Could you check a few things on this drawing? It's one solid part, dimensions in mm from its lowest x, y, z. A direction names the side the tool comes from. Round coordinates to 2 decimals unless told otherwise and drop trailing zeros. Loops run counter-clockwise (first coordinate to the right, second up) from the corner with the lowest first, then second, coordinate; pieces in that order, holes last. Notation, with made-up numbers: (9.25, 29) -> (54.25, 29) arc R12 ccw to (54.25, 50) -> close; hole circle Ø6 at (18, -11). An arc over 180 degrees is marked (long way). Put each result on its own line as item: value. Start each with the question number.
1. Imagine slicing it at A-A, the plane y = 44.5. Please give me the cut outline in (x, z), and give its area (3 significant figures).
2. I need wall thicknesses on line 1 (Y direction, x = 4.75, z = 10); line 2 (Z direction, x = 6.75, y = 17); line 3 (X direction, y = 20, z = 9). Which ranges of each line are inside material? Lowest first, please. Write a range as [from, to].
3. Which directions (+Z, -Z, +X, -X, +Y, -Y) give clear straight access to the entire face, cutting with the end or side of a thin tool? Please do the marked faces 1 and 2.
4. I'm going to push flat-ended pins straight in: P1, Ø3, axis at x = 12.5, y = 25, coming from the +Z side; P2, Ø6.5, axis at x = 8.5, z = 4, coming from the -Y side; P3, Ø2, axis at y = 10, z = 9.5, coming from the +X side; P4, Ø1, axis at x = 12, z = 4.5, coming from the -Y side. Where does each tip first touch, or does it pass through?
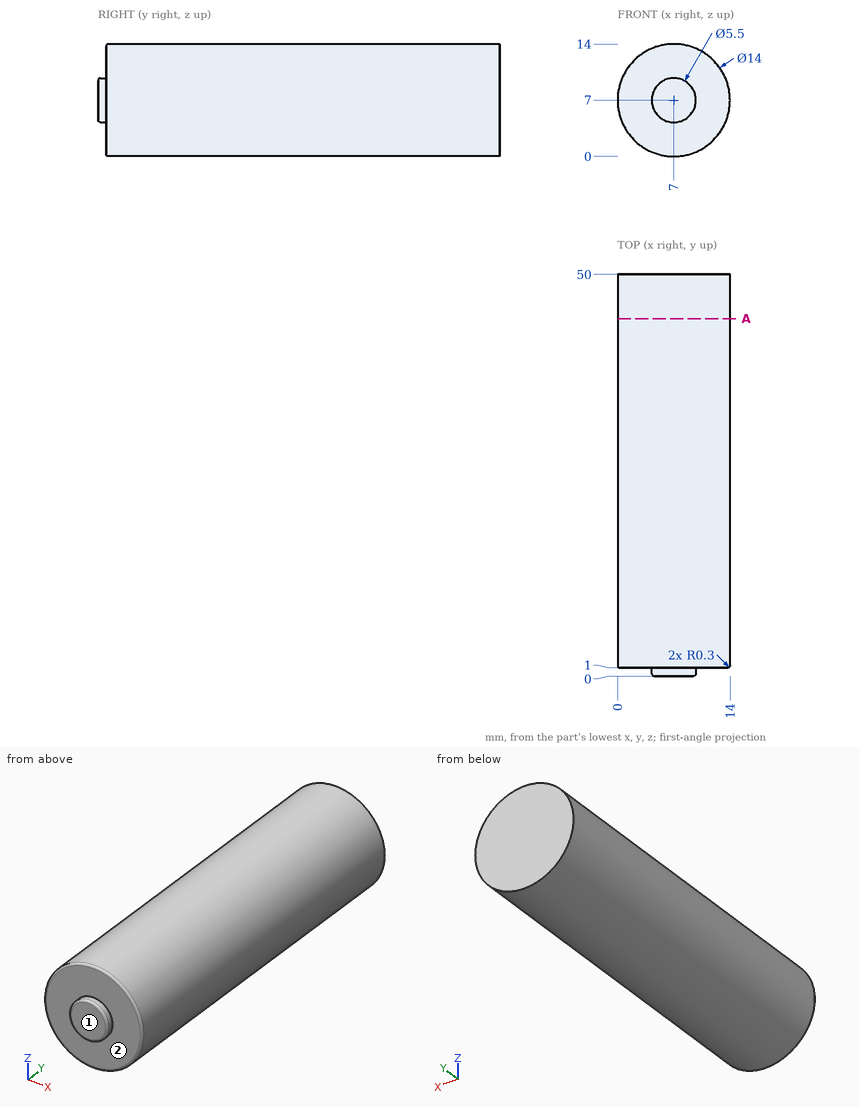
Entries:
1. outline: circle Ø14 at (7, 7)
1. area: 154 mm^2
2. line 1: [1, 50]
2. line 2: [0, 14]
2. line 3: [0.29, 13.71]
3. face 1: +Z, -Z, +X, -X, -Y
3. face 2: -Y
4. P1: z = 12.74
4. P2: y = 0
4. P3: x = 13.84
4. P4: y = 1
